Here's how the part is built. I have some questions about the finished solid (model axes, mm). Give positions to 0.01 mm unless a question says otherwise; leave off trailing zeros. Loops run counter-clockwise (first coordinate to the right, second up) from the corner with the lowest first, then second, coordinate; pieces in that order, holes last. Notation, with made-up numbers: (77.25, 37) - (103.25, 37) arc R30 cw to (103.25, 72) - close; hole circle Ø7 at (26.5, 10). An arc over 180 degrees is marked (long way). One line per item, written item: value. Start each with the question number.
```python
from build123d import *

# Parameters (mm, degrees)
SKETCH1_R               = 12.192
SKETCH1_R_2             = 9.652
MAIN_INNER_TUBE_DEPTH   = 135.89
SKETCH2_W               = 24.384
SKETCH2_H               = 24.384
SKETCH2_R               = 9.652
RECTANGLE_OUTSIDE_DEPTH = 135.89


with BuildPart() as part:
    # Sketch1 → Main Inner Tube (new body)
    with BuildSketch(Plane.XY):
        Circle(SKETCH1_R)
        Circle(SKETCH1_R_2, mode=Mode.SUBTRACT)
    extrude(amount=MAIN_INNER_TUBE_DEPTH)

    # Sketch2 → Rectangle Outside (add, through all)
    with BuildSketch(Plane(origin=(0, 0, 0), x_dir=(-1, 0, 0), z_dir=(0, 0, -1))):
        Rectangle(SKETCH2_W, SKETCH2_H)
        with Locations(Location((0, 0, 0), (0, 0, 180))):
            Circle(SKETCH2_R, mode=Mode.SUBTRACT)
    extrude(amount=-RECTANGLE_OUTSIDE_DEPTH)


solid = part.part
```
(1) If we section it at A-A on x = 0: List the corners of the cut face in (y, z) for me, plus the area to 3 significant figures.
(2) If we mould it in two halves opening along Z, with no side actions, what happens to faces 1 (the face through (-7.66, -5.87, 66.99)), 2 (the face through (8, 6, 0)), 3 (the face through (8, 6, 135.89))? For each: pulls with the +Z half, pulls with the -Z half, needs draft (parallel to the pull), parting line crosses it, or undercut.
(3) If we section it at C-C on z = 42.5: List the corners of the cut face in (x, y) for me.
(4) If we section it at B-B on y = -8: List the corners of the cut face in (x, z) for me.
(5) Please list where these lines run through material, in increasing order: probe 1 along Y at (x, z) = (0, 49); probe 2 along Y at (x, z) = (0.5, 13.5); probe 3 along X at (y, z) = (8.5, 27). Write a range as from..to.
Found:
1. outline: (-12.19, 0) - (-9.65, 0) - (-9.65, 135.89) - (-12.19, 135.89) - close; (9.65, 0) - (12.19, 0) - (12.19, 135.89) - (9.65, 135.89) - close
1. area: 690 mm^2
2. face 1: needs draft
2. face 2: pulls with the -Z half
2. face 3: pulls with the +Z half
3. outline: (-12.19, -12.19) - (12.19, -12.19) - (12.19, 12.19) - (-12.19, 12.19) - close; hole circle Ø19.3 at (0, 0)
4. outline: (-12.19, 0) - (-5.4, 0) - (-5.4, 135.89) - (-12.19, 135.89) - close; (5.4, 0) - (12.19, 0) - (12.19, 135.89) - (5.4, 135.89) - close
5. probe 1: -12.19..-9.65, 9.65..12.19
5. probe 2: -12.19..-9.64, 9.64..12.19
5. probe 3: -12.19..-4.57, 4.57..12.19
